Autodesk Inventor part; units mm, degrees
ref_plane "YZ Plane" through (0, 0, 0) normal (1, 0, 0) x (0, 1, 0)
ref_plane "XZ Plane" through (0, 0, 0) normal (0, 1, 0) x (-1, 0, 0)
ref_plane "XY Plane" through (0, 0, 0) normal (0, 0, 1) x (1, 0, 0)
sketch "Sketch1" plane through (0, 0, 0) normal (0, 1, 0) x (-1, 0, 0)
  line L0 (0, 0) -> (-25.4, 0)
  line L1 (-25.4, 0) -> (-25.4, -25.4)
  line L2 (-25.4, -25.4) -> (0, -25.4)
  line L3 (0, -25.4) -> (0, 0)
  dimension "d0" = 25.4
  dimension "d1" = 25.4
extrude "Extrusion1" add sketch "Sketch1" along normal blind 307.975
sketch "Sketch4" plane through (0, 0, 0) normal (0, -1, 0) x (1, 0, 0)
  line L0 (22.86, -2.54) -> (2.54, -2.54)
  line L1 (2.54, -2.54) -> (2.54, -22.86)
  line L2 (2.54, -22.86) -> (22.86, -22.86)
  line L3 (22.86, -22.86) -> (22.86, -2.54)
  line L4 (25.4, 0) -> (25.4, -25.4)
  line L5 (25.4, -25.4) -> (0, -25.4)
  point P0 (0, 0)
  dimension "d13" = 20.32
  dimension "d14" = 20.32
  dimension "d15" = 2.54
  dimension "d16" = 2.54
extrude "Extrusion4" cut sketch "Sketch4" against normal blind 448.31
sketch "Sketch15" plane through (0, 0, -25.4) normal (-1, 0, 0) x (0, 0, 1)
  point P0 (25.4, 0)
properties part number "Control Panel Mount"
Can you work these out from the model? Positions are in its coordinate system, mm. A direction names the side the tool comes from. Give positions to 0.01 mm unless a question says otherwise; leave off trailing zeros. Write each loop counter-clockwise with the first axis right and the second up, starting at its lowest first coordinate (ties: lowest second). Pieces come first, ordered by that corner, then holes. Notation, with made-up numbers: (47, -20.5) -> (101, -20.5) arc R20 cw to (101, -9.5) -> close; hole circle Ø11 at (-3.5, 18). An arc over 180 degrees is marked (long way). One line per item, written item: value.
Q1. We'd pull the mould along Z, two halves only. Please class faces 3 (the face through (0, 152, -13)), 4 (the face through (2.54, 152, -13)), 5 (the face through (13, 152, 0)): +Z half, -Z half, draft (parallel to the pull), parting line (faces both ways), or undercut.
Results found:
face 3: draft
face 4: undercut
face 5: +Z half
Q2. Imagine slicing it at A-A on x = 8. Please give me the cut outline in (y, z) (3 decimals), and give its area (3 significant figures).
Results found:
outline: (0, -25.4) -> (307.975, -25.4) -> (307.975, -22.86) -> (0, -22.86) -> close; (0, -2.54) -> (307.975, -2.54) -> (307.975, 0) -> (0, 0) -> close
area: 1,560 mm^2
Q3. Imagine slicing it at C-C on y = 140.5. Please give me the cut outline in (x, z).
Results found:
outline: (0, -25.4) -> (25.4, -25.4) -> (25.4, 0) -> (0, 0) -> close; hole (2.54, -22.86) -> (22.86, -22.86) -> (22.86, -2.54) -> (2.54, -2.54) -> close
Q4. Imagine slicing it at B-B on z = -9. Please give me the cut outline in (x, y) (3 decimals).
Results found:
outline: (0, 0) -> (2.54, 0) -> (2.54, 307.975) -> (0, 307.975) -> close; (22.86, 0) -> (25.4, 0) -> (25.4, 307.975) -> (22.86, 307.975) -> close
Q5. For P1, Ø5, axis at y = 32, z = -4.5, coming from the -X side, with a flat end and sliding along its axis, tell me the tip position at first contact or that it passes through.
Results found:
P1: stops at x = 0
Q6. Please list where these lines run through material, in increasing order: line 1 (X direction, y = 114, z = -3.5); line 2 (Z direction, x = 5, y = 62.5). Write a range as [from, to].
Results found:
line 1: x = [0, 2.54], [22.86, 25.4]
line 2: z = [-25.4, -22.86], [-2.54, 0]
Q7. Which directions (+Z, -Z, +X, -X, +Y, -Y) give clear straight access to the entire face, cutting with the end or side of a thin tool? Please do faces 1 (the face through (13, 152, -25.4)), 2 (the face through (22.86, 152, -13)).
Results found:
face 1: -Z, +X, -X, +Y, -Y
face 2: +Y, -Y
